```python
from build123d import *

# Parameters (mm, degrees)
SKETCH_2_W      = 156
SKETCH_2_H      = 115
SKETCH_2_W_2    = 110
SKETCH_2_H_2    = 16
EXTRUDE_1_DEPTH = 3
SKETCH_1_W      = 150
SKETCH_1_H      = 110
SKETCH_1_W_2    = 144
SKETCH_1_H_2    = 104
EXTRUDE_2_DEPTH = 2
SKETCH_3_R      = 2.5
EXTRUDE_3_DEPTH = 28.3
SKETCH_5_R      = 1.25
EXTRUDE_4_DEPTH = 1.7


with BuildPart() as part:
    # 草图2 → 凸台-拉伸1 (new body)
    with BuildSketch(Plane.XY.offset(-2003.6216566)):
        with Locations((145.628836913, 15.276761468)):
            Rectangle(SKETCH_2_W, SKETCH_2_H)
        with Locations((145.628836913, 0.776761468)):
            Rectangle(SKETCH_2_W_2, SKETCH_2_H_2, mode=Mode.SUBTRACT)
        with BuildLine():
            Line((89.628836913, 35.776761468), (89.628836913, 55.776761468))
            ThreePointArc((89.628836913, 55.776761468), (90.628836913, 56.776761468), (91.628836913, 55.776761468))
            Line((91.628836913, 55.776761468), (91.628836913, 35.776761468))
            ThreePointArc((91.628836913, 35.776761468), (90.628836913, 34.776761468), (89.628836913, 35.776761468))
        make_face(mode=Mode.SUBTRACT)
        with BuildLine():
            Line((95.628836913, 35.776761468), (95.628836913, 55.776761468))
            ThreePointArc((95.628836913, 55.776761468), (96.628836913, 56.776761468), (97.628836913, 55.776761468))
            Line((97.628836913, 55.776761468), (97.628836913, 35.776761468))
            ThreePointArc((97.628836913, 35.776761468), (96.628836913, 34.776761468), (95.628836913, 35.776761468))
        make_face(mode=Mode.SUBTRACT)
        with BuildLine():
            Line((101.628836913, 35.776761468), (101.628836913, 55.776761468))
            ThreePointArc((101.628836913, 55.776761468), (102.628836913, 56.776761468), (103.628836913, 55.776761468))
            Line((103.628836913, 55.776761468), (103.628836913, 35.776761468))
            ThreePointArc((103.628836913, 35.776761468), (102.628836913, 34.776761468), (101.628836913, 35.776761468))
        make_face(mode=Mode.SUBTRACT)
        with BuildLine():
            Line((107.628836913, 35.776761468), (107.628836913, 55.776761468))
            ThreePointArc((107.628836913, 55.776761468), (108.628836913, 56.776761468), (109.628836913, 55.776761468))
            Line((109.628836913, 55.776761468), (109.628836913, 35.776761468))
            ThreePointArc((109.628836913, 35.776761468), (108.628836913, 34.776761468), (107.628836913, 35.776761468))
        make_face(mode=Mode.SUBTRACT)
        with BuildLine():
            Line((113.628836913, 35.776761468), (113.628836913, 55.776761468))
            ThreePointArc((113.628836913, 55.776761468), (114.628836913, 56.776761468), (115.628836913, 55.776761468))
            Line((115.628836913, 55.776761468), (115.628836913, 35.776761468))
            ThreePointArc((115.628836913, 35.776761468), (114.628836913, 34.776761468), (113.628836913, 35.776761468))
        make_face(mode=Mode.SUBTRACT)
        with BuildLine():
            Line((119.628836913, 35.776761468), (119.628836913, 55.776761468))
            ThreePointArc((119.628836913, 55.776761468), (120.628836913, 56.776761468), (121.628836913, 55.776761468))
            Line((121.628836913, 55.776761468), (121.628836913, 35.776761468))
            ThreePointArc((121.628836913, 35.776761468), (120.628836913, 34.776761468), (119.628836913, 35.776761468))
        make_face(mode=Mode.SUBTRACT)
        with BuildLine():
            Line((125.628836913, 35.776761468), (125.628836913, 55.776761468))
            ThreePointArc((125.628836913, 55.776761468), (126.628836913, 56.776761468), (127.628836913, 55.776761468))
            Line((127.628836913, 55.776761468), (127.628836913, 35.776761468))
            ThreePointArc((127.628836913, 35.776761468), (126.628836913, 34.776761468), (125.628836913, 35.776761468))
        make_face(mode=Mode.SUBTRACT)
        with BuildLine():
            Line((131.628836913, 35.776761468), (131.628836913, 55.776761468))
            ThreePointArc((131.628836913, 55.776761468), (132.628836913, 56.776761468), (133.628836913, 55.776761468))
            Line((133.628836913, 55.776761468), (133.628836913, 35.776761468))
            ThreePointArc((133.628836913, 35.776761468), (132.628836913, 34.776761468), (131.628836913, 35.776761468))
        make_face(mode=Mode.SUBTRACT)
        with BuildLine():
            Line((137.628836913, 35.776761468), (137.628836913, 55.776761468))
            ThreePointArc((137.628836913, 55.776761468), (138.628836913, 56.776761468), (139.628836913, 55.776761468))
            Line((139.628836913, 55.776761468), (139.628836913, 35.776761468))
            ThreePointArc((139.628836913, 35.776761468), (138.628836913, 34.776761468), (137.628836913, 35.776761468))
        make_face(mode=Mode.SUBTRACT)
        with BuildLine():
            Line((143.628836913, 35.776761468), (143.628836913, 55.776761468))
            ThreePointArc((143.628836913, 55.776761468), (144.628836913, 56.776761468), (145.628836913, 55.776761468))
            Line((145.628836913, 55.776761468), (145.628836913, 35.776761468))
            ThreePointArc((145.628836913, 35.776761468), (144.628836913, 34.776761468), (143.628836913, 35.776761468))
        make_face(mode=Mode.SUBTRACT)
        with BuildLine():
            Line((149.628836913, 35.776761468), (149.628836913, 55.776761468))
            ThreePointArc((149.628836913, 55.776761468), (150.628836913, 56.776761468), (151.628836913, 55.776761468))
            Line((151.628836913, 55.776761468), (151.628836913, 35.776761468))
            ThreePointArc((151.628836913, 35.776761468), (150.628836913, 34.776761468), (149.628836913, 35.776761468))
        make_face(mode=Mode.SUBTRACT)
        with BuildLine():
            Line((155.628836913, 35.776761468), (155.628836913, 55.776761468))
            ThreePointArc((155.628836913, 55.776761468), (156.628836913, 56.776761468), (157.628836913, 55.776761468))
            Line((157.628836913, 55.776761468), (157.628836913, 35.776761468))
            ThreePointArc((157.628836913, 35.776761468), (156.628836913, 34.776761468), (155.628836913, 35.776761468))
        make_face(mode=Mode.SUBTRACT)
        with BuildLine():
            Line((161.628836913, 35.776761468), (161.628836913, 55.776761468))
            ThreePointArc((161.628836913, 55.776761468), (162.628836913, 56.776761468), (163.628836913, 55.776761468))
            Line((163.628836913, 55.776761468), (163.628836913, 35.776761468))
            ThreePointArc((163.628836913, 35.776761468), (162.628836913, 34.776761468), (161.628836913, 35.776761468))
        make_face(mode=Mode.SUBTRACT)
        with BuildLine():
            Line((167.628836913, 35.776761468), (167.628836913, 55.776761468))
            ThreePointArc((167.628836913, 55.776761468), (168.628836913, 56.776761468), (169.628836913, 55.776761468))
            Line((169.628836913, 55.776761468), (169.628836913, 35.776761468))
            ThreePointArc((169.628836913, 35.776761468), (168.628836913, 34.776761468), (167.628836913, 35.776761468))
        make_face(mode=Mode.SUBTRACT)
        with BuildLine():
            Line((173.628836913, 35.776761468), (173.628836913, 55.776761468))
            ThreePointArc((173.628836913, 55.776761468), (174.628836913, 56.776761468), (175.628836913, 55.776761468))
            Line((175.628836913, 55.776761468), (175.628836913, 35.776761468))
            ThreePointArc((175.628836913, 35.776761468), (174.628836913, 34.776761468), (173.628836913, 35.776761468))
        make_face(mode=Mode.SUBTRACT)
        with BuildLine():
            Line((179.628836913, 35.776761468), (179.628836913, 55.776761468))
            ThreePointArc((179.628836913, 55.776761468), (180.628836913, 56.776761468), (181.628836913, 55.776761468))
            Line((181.628836913, 55.776761468), (181.628836913, 35.776761468))
            ThreePointArc((181.628836913, 35.776761468), (180.628836913, 34.776761468), (179.628836913, 35.776761468))
        make_face(mode=Mode.SUBTRACT)
        with BuildLine():
            Line((185.628836913, 35.776761468), (185.628836913, 55.776761468))
            ThreePointArc((185.628836913, 55.776761468), (186.628836913, 56.776761468), (187.628836913, 55.776761468))
            Line((187.628836913, 55.776761468), (187.628836913, 35.776761468))
            ThreePointArc((187.628836913, 35.776761468), (186.628836913, 34.776761468), (185.628836913, 35.776761468))
        make_face(mode=Mode.SUBTRACT)
        with BuildLine():
            Line((191.628836913, 35.776761468), (191.628836913, 55.776761468))
            ThreePointArc((191.628836913, 55.776761468), (192.628836913, 56.776761468), (193.628836913, 55.776761468))
            Line((193.628836913, 55.776761468), (193.628836913, 35.776761468))
            ThreePointArc((193.628836913, 35.776761468), (192.628836913, 34.776761468), (191.628836913, 35.776761468))
        make_face(mode=Mode.SUBTRACT)
        with BuildLine():
            Line((197.628836913, 35.776761468), (197.628836913, 55.776761468))
            ThreePointArc((197.628836913, 55.776761468), (198.628836913, 56.776761468), (199.628836913, 55.776761468))
            Line((199.628836913, 55.776761468), (199.628836913, 35.776761468))
            ThreePointArc((199.628836913, 35.776761468), (198.628836913, 34.776761468), (197.628836913, 35.776761468))
        make_face(mode=Mode.SUBTRACT)
        with BuildLine():
            Line((203.628836913, 35.776761468), (203.628836913, 55.776761468))
            ThreePointArc((203.628836913, 55.776761468), (204.628836913, 56.776761468), (205.628836913, 55.776761468))
            Line((205.628836913, 55.776761468), (205.628836913, 35.776761468))
            ThreePointArc((205.628836913, 35.776761468), (204.628836913, 34.776761468), (203.628836913, 35.776761468))
        make_face(mode=Mode.SUBTRACT)
    extrude(amount=EXTRUDE_1_DEPTH)

    # 草图1 → 凸台-拉伸2 (add)
    with BuildSketch(Plane.XY.offset(-2003.6216566)):
        with Locations((145.628836913, 15.776761468)):
            Rectangle(SKETCH_1_W, SKETCH_1_H)
        with Locations((145.628836913, 15.776761468)):
            Rectangle(SKETCH_1_W_2, SKETCH_1_H_2, mode=Mode.SUBTRACT)
    extrude(amount=-EXTRUDE_2_DEPTH)

    # 草图3 → 凸台-拉伸3 (add)
    with BuildSketch(Plane(origin=(0, 0, -2003.6216566), x_dir=(-1, 0, 0), z_dir=(0, 0, -1))):
        with Locations(Location((-196.628836913, 65.776761468, 0), (0, 0, 126.869897646))):
            Circle(SKETCH_3_R)
        with Locations(Location((-94.628836913, 65.776761468, 0), (0, 0, 126.869897646))):
            Circle(SKETCH_3_R)
        with Locations(Location((-94.628836913, -10.223238532, 0), (0, 0, 180))):
            Circle(SKETCH_3_R)
        with Locations(Location((-196.628836913, -10.223238532, 0), (0, 0, 180))):
            Circle(SKETCH_3_R)
    extrude(amount=EXTRUDE_3_DEPTH)

    # 草图5 → 凸台-拉伸4 (add)
    with BuildSketch(Plane(origin=(0, 0, -2031.9216566), x_dir=(-1, 0, 0), z_dir=(0, 0, -1))):
        with Locations((-196.628836913, 65.776761468)):
            Circle(SKETCH_5_R)
        with Locations((-94.628836913, 65.776761468)):
            Circle(SKETCH_5_R)
        with Locations((-94.628836913, -10.223238532)):
            Circle(SKETCH_5_R)
        with Locations((-196.628836913, -10.223238532)):
            Circle(SKETCH_5_R)
    extrude(amount=EXTRUDE_4_DEPTH)


solid = part.part
```
For this review, take the finished solid that the model builds, in its own axes (mm). A direction names the side the tool comes from. Round coordinates to 2 decimals unless told otherwise and drop trailing zeros. Write each loop counter-clockwise with the first axis right and the second up, starting at its lowest first coordinate (ties: lowest second). Pieces come first, ordered by that corner, then holes. Notation, with made-up numbers: (20.5, 22) - (48.5, 22) arc R17 ccw to (48.5, 51) - close; hole circle Ø7 at (45.25, 44.25). An arc over 180 degrees is marked (long way). Answer as CSV lines item,"result". Start each with the question number.
(1) Add section A-A, the plane y = 1. State the section outline as (x, z) points, plus the area to 3 significant figures.
(2) Add section C-C, the plane z = -2019. State the section outline as (x, y) points, plus the area to 3 significant figures.
(3) Add section B-B, the plane y = -22. State the section outline as (x, z) points.
(4) Machinability: for faces 5 (the flat face through (67.629, 14, -2002)), 6 (the flat face through (185.629, 46, -2002)), 7 (the flat face through (145, 17, -2003.622)), which of the approach directions +Z, -Z, +X, -X, +Y, -Y give a long, thin tool a straight path to every point of the face, cutting with its end or side? Answer none if there is none.
(5) For line 1 (X direction, y = -12, z = -2005); line 2 (Z direction, x = 151, y = 61.5); line 3 (Y direction, x = 123, z = -2005), list the stretches that pass through material, from the lowest coordinate up.
(6) Mouldability with a two-part tool opening along X and no side actions: class faces 1 (the flat face through (145, -42.223, -2002)), 2 (the flat face through (115.629, 46, -2002)), 3 (the flat face through (121.629, 46, -2002)), 4 (the flat face through (223.629, 14, -2002)) as +X half, -X half, draft (parallel to the pull), parting line (faces both ways), or undercut.
(7) For pin 1 (1.5 mm diameter, centred on x = 98.5, z = -2005.5, fed in from +Y); pin 2 (2 mm diameter, centred on x = 139.5, z = -2004, fed in from +Y); pin 3 (6 mm diameter, centred on x = 191.5, z = -2010.5, fed in from -Y); pin 4 (12 mm diameter, centred on x = 178.5, z = -2015.5, fed in from +Y), all flat-tipped, find the tip position at first contact; note any pin that passes through.
(8) Add section D-D, the plane y = 46. State how many separate pieces and enclosed holes the cut face has, plus the area to 3 significant figures.
From the geometry:
1,outline,"(67.63, -2003.62) - (70.63, -2003.62) - (70.63, -2005.62) - (73.63, -2005.62) - (73.63, -2003.62) - (90.63, -2003.62) - (90.63, -2000.62) - (67.63, -2000.62) - close; (200.63, -2003.62) - (217.63, -2003.62) - (217.63, -2005.62) - (220.63, -2005.62) - (220.63, -2003.62) - (223.63, -2003.62) - (223.63, -2000.62) - (200.63, -2000.62) - close"
1,area,"150 mm²"
2,outline,"circle Ø5 at (94.63, -10.22); circle Ø5 at (94.63, 65.78); circle Ø5 at (196.63, -10.22); circle Ø5 at (196.63, 65.78)"
2,area,"78.5 mm²"
3,outline,"(67.63, -2003.62) - (70.63, -2003.62) - (70.63, -2005.62) - (73.63, -2005.62) - (73.63, -2003.62) - (217.63, -2003.62) - (217.63, -2005.62) - (220.63, -2005.62) - (220.63, -2003.62) - (223.63, -2003.62) - (223.63, -2000.62) - (67.63, -2000.62) - close"
4,face 5,"+Z, -Z, -X, +Y, -Y"
4,face 6,"+Z, -Z"
4,face 7,"-Z"
5,line 1,"x = 70.63 to 73.63, 92.87 to 96.39, 194.87 to 198.39, 217.63 to 220.63"
5,line 2,"z = -2003.62 to -2000.62"
5,line 3,"y = -39.22 to -36.22, 67.78 to 70.78"
6,face 1,"draft"
6,face 2,"undercut"
6,face 3,"undercut"
6,face 4,"+X half"
7,pin 1,"stops at y = 70.78"
7,pin 2,"stops at y = 72.78"
7,pin 3,"stops at y = -11.53"
7,pin 4,"passes through"
8,separate pieces,"21"
8,enclosed holes,"0"
8,area,"360 mm²"
